Design review of the part built by this model. Coordinates are the model's own, in mm. Round coordinates to 2 decimals unless told otherwise and drop trailing zeros. Write each loop counter-clockwise with the first axis right and the second up, starting at its lowest first coordinate (ties: lowest second). Pieces come first, ordered by that corner, then holes. Notation, with made-up numbers: (55, 24) -> (103, 24) arc R14 cw to (103, 50) -> close; hole circle Ø9 at (4.25, 84). An arc over 180 degrees is marked (long way). One line per question, with ' | ' between items. Start each with the question number.
1) For probe 1 along X at (y, z) = (0.5, -58.42); probe 2 along X at (y, z) = (0.5, -50.8); probe 3 along Z at (x, y) = (38, 0.95), list the stretches that pass through material, from the lowest coordinate up.
2) Consider section A-A (z = -2.54). Give the boundary of the cut face in (x, y), then the cut area to 3 significant figures.
3) Insertion check: pin 1 Ø1.1 at (x, z) = (2.5, -10) entering from -Y. The pin has a flat end and moves straight along its axis. Give the tip position at first contact, or say it passes through.
```python
from build123d import *

# Parameters (mm, degrees)
SKETCH1_W           = 40.64
SKETCH1_H           = 60.96
SKETCH1_R           = 1
SKETCH1_R_2         = 0.5
BOSS_EXTRUDE1_DEPTH = 1.5
SKETCH1_5_R         = 0.5
CUT_EXTRUDE1_DEPTH  = 0.75


with BuildPart() as part:
    # Sketch1 → Boss-Extrude1 (new body)
    with BuildSketch(Plane(origin=(0, 0, 0), x_dir=(1, 0, 0), z_dir=(0, 1, 0))):
        with Locations((20.32, 30.48)):
            Rectangle(SKETCH1_W, SKETCH1_H)
        with Locations(Location((38.1, 58.42, 0), (0, 0, 270))):  # turned: the seam where the file's is
            Circle(SKETCH1_R, mode=Mode.SUBTRACT)
        with Locations((38.1, 50.8)):
            Circle(SKETCH1_R_2, mode=Mode.SUBTRACT)
        with Locations(Location((38.1, 2.54, 0), (0, 0, 270))):  # turned: the seam where the file's is
            Circle(SKETCH1_R, mode=Mode.SUBTRACT)
        with Locations(Location((2.54, 58.42, 0), (0, 0, 270))):  # turned: the seam where the file's is
            Circle(SKETCH1_R, mode=Mode.SUBTRACT)
        with Locations((2.54, 10.16)):
            Circle(SKETCH1_R_2, mode=Mode.SUBTRACT)
        with Locations(Location((2.54, 2.54, 0), (0, 0, 270))):  # turned: the seam where the file's is
            Circle(SKETCH1_R, mode=Mode.SUBTRACT)
        with Locations((2.54, 50.8)):
            Circle(SKETCH1_R_2, mode=Mode.SUBTRACT)
        with Locations((38.1, 10.16)):
            Circle(SKETCH1_R_2, mode=Mode.SUBTRACT)
        with Locations((2.54, 10.16)):
            Circle(SKETCH1_R_2)
        with Locations((38.1, 10.16)):
            Circle(SKETCH1_R_2)
        with Locations((38.1, 50.8)):
            Circle(SKETCH1_R_2)
        with Locations((2.54, 50.8)):
            Circle(SKETCH1_R_2)
    extrude(amount=BOSS_EXTRUDE1_DEPTH)

    # Sketch1_5 → Cut-Extrude1 (cut)
    with BuildSketch(Plane(origin=(0, 0, 0), x_dir=(1, 0, 0), z_dir=(0, 1, 0))):
        with Locations(Location((2.54, 50.8, 0), (0, 0, 270))):  # turned: the seam where the file's is
            Circle(SKETCH1_5_R)
        with Locations(Location((38.1, 50.8, 0), (0, 0, 270))):  # turned: the seam where the file's is
            Circle(SKETCH1_5_R)
        with Locations(Location((38.1, 10.16, 0), (0, 0, 270))):  # turned: the seam where the file's is
            Circle(SKETCH1_5_R)
        with Locations(Location((2.54, 10.16, 0), (0, 0, 270))):  # turned: the seam where the file's is
            Circle(SKETCH1_5_R)
    extrude(amount=CUT_EXTRUDE1_DEPTH, mode=Mode.SUBTRACT)


solid = part.part
```
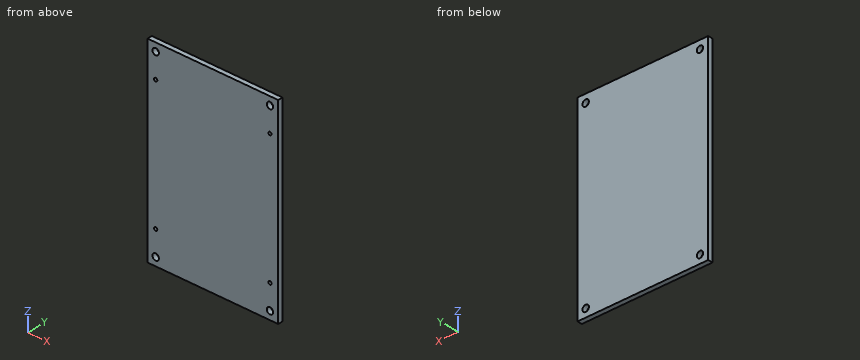
From the geometry:
1) probe 1: x = 0 to 1.54, 3.54 to 37.1, 39.1 to 40.64 | probe 2: x = 0 to 2.04, 3.04 to 37.6, 38.6 to 40.64 | probe 3: z = -60.96 to -59.41, -57.43 to -3.53, -1.55 to 0
2) outline: (0, 0) -> (1.54, 0) -> (1.54, 1.5) -> (0, 1.5) -> close; (3.54, 0) -> (37.1, 0) -> (37.1, 1.5) -> (3.54, 1.5) -> close; (39.1, 0) -> (40.64, 0) -> (40.64, 1.5) -> (39.1, 1.5) -> close | area: 55.0 mm2
3) pin 1: stops at y = 0
